Geometry check sheet. Reference: the model listing, model coordinates, mm. Face numbers are marked on the shaded views. Give positions to 0.01 mm unless a question says otherwise; leave off trailing zeros. Write item = value, one per line. Start each with the question number.
1. Thickness scan on line 1 along Y through (x, z) = (31, 17); line 2 along X through (y, z) = (4, 17); line 3 along X through (y, z) = (1, -20.5). Record the ranges inside material, lowest first.
2. Mould release check, pull along Z, two halves, no side actions. Record for the marked faces 1 and 2: pulls with the +Z half, pulls with the -Z half, needs draft (parallel to the pull), parting line crosses it, or undercut.
3. Depth check by flat-ended pin: P1, Ø3, axis at y = 20.5, z = -8, coming from the -X side; P2, Ø1.5, axis at y = -5.5, z = -2, coming from the +X side; P3, Ø6, axis at x = 25.5, z = 7, coming from the +Y side. Enter the tip coordinate at first touch or a pass-through.
Autodesk Inventor part; units mm, degrees
ref_plane "YZ Plane" through (0, 0, 0) normal (1, 0, 0) x (0, 1, 0)
ref_plane "XZ Plane" through (0, 0, 0) normal (0, 1, 0) x (-1, 0, 0)
ref_plane "XY Plane" through (0, 0, 0) normal (0, 0, 1) x (1, 0, 0)
sketch "Sketch1" plane through (0, 0, 0) normal (0, 0, 1) x (1, 0, 0)
  line L0 (13.0382, 19.2392) -> (29.1292, 26.2353)
  line L1 (29.1292, 26.2353) -> (45.6654, 22.7373)
  line L2 (45.6654, 22.7373) -> (48.273, 12.4976)
  line L3 (48.273, 12.4976) -> (54.5695, 23.1189)
  line L4 (54.5695, 23.1189) -> (59.8483, 17.6174)
  line L5 (59.8483, 17.6174) -> (48.273, -2.7666)
  line L6 (48.273, -2.7666) -> (13.0382, 19.2392)
  line L7 (11.0461, 18.3731) -> (46.9692, -5.0626) construction
  point P0 (0, 0)
revolve "Revolution1" add sketch "Sketch1" angle 360 about axis through (11.0461, 18.3731, 0) along (0.8375, -0.5464, 0)
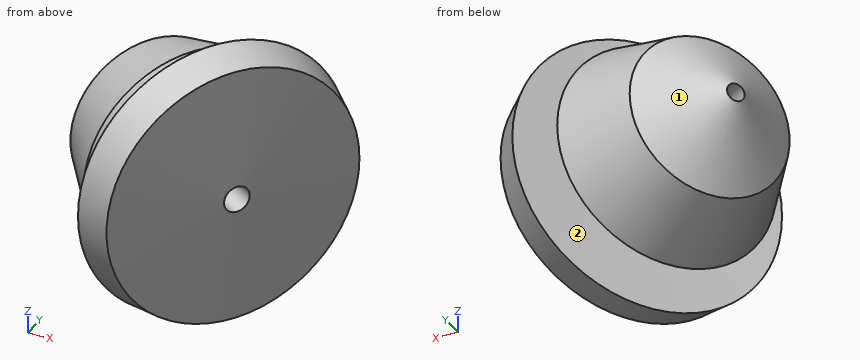
Answers:
q1.line_1 = -19.57 to -13.37, -5.94 to 16.07
q1.line_2 = 20.43 to 40.12, 42.61 to 51.43
q1.line_3 = 27.42 to 34.05, 40.51 to 49.34
q2.face_1 = parting line crosses it
q2.face_2 = undercut
q3.P1 = 18.38
q3.P2 = 46.75
q3.P3 = 25.21
